```python
from build123d import *

# Parameters (mm, degrees)
SKETCH1_W           = 310
SKETCH1_H           = 120
SKETCH1_R           = 2.5
BOSS_EXTRUDE1_DEPTH = 3
CUT_EXTRUDE1_REACH  = 168.235
SKETCH2_R           = 12.5


with BuildPart() as part:
    # Sketch1 → Boss-Extrude1 (new body)
    with BuildSketch(Plane(origin=(0, 0, 0), x_dir=(1, 0, 0), z_dir=(0, 1, 0))):
        Rectangle(SKETCH1_W, SKETCH1_H)
        with Locations(Location((-125, 47, 0), (0, 0, 270))):
            Circle(SKETCH1_R, mode=Mode.SUBTRACT)
        with Locations(Location((125, 47, 0), (0, 0, 90))):
            Circle(SKETCH1_R, mode=Mode.SUBTRACT)
        with Locations(Location((125, -47, 0), (0, 0, 270))):
            Circle(SKETCH1_R, mode=Mode.SUBTRACT)
        with Locations(Location((-125, -47, 0), (0, 0, 90))):
            Circle(SKETCH1_R, mode=Mode.SUBTRACT)
    extrude(amount=BOSS_EXTRUDE1_DEPTH)

    # Sketch2 → Cut-Extrude1 (cut, up to next)
    with BuildSketch(Plane.XZ, mode=Mode.PRIVATE) as cut_extrude1_sk1:
        with Locations((155, -20)):
            Circle(SKETCH2_R)
    cut_extrude1_tool1 = extrude(cut_extrude1_sk1.sketch, amount=-CUT_EXTRUDE1_REACH, mode=Mode.PRIVATE) & part.part
    add(cut_extrude1_tool1.solids().sort_by_distance((155, 0, -20))[0], mode=Mode.SUBTRACT)


solid = part.part
```
Model file for the job. Use its own axes, mm. Give positions to 0.01 mm unless a question says otherwise; leave off trailing zeros. Loops run counter-clockwise (first coordinate to the right, second up) from the corner with the lowest first, then second, coordinate; pieces in that order, holes last. Notation, with made-up numbers: (-12.5, 65.5) -> (25.5, 65.5) arc R18 cw to (25.5, 83.5) -> close; hole circle Ø8 at (18.5, 55). An arc over 180 degrees is marked (long way). Use CSV: the item, a comma, the result in double quotes. Start each with the question number.
1) Mould opens along Z. For faces 1 (the cylindrical face through (-122.52, 1.48, -47.33)), 2 (the flat face through (-2, 0, -1)) say: released by +Z, released by -Z, zero draft, split by the parting line, or undercut.
2) Flat gauge pins, fed straight in: pin 1 Ø8 at (x, z) = (125, -47) entering from -Y; pin 2 Ø4.5 at (x, z) = (-125, 47) entering from +Y. Where does each tip first touch, or does it go through?
3) Slice it at A-A on z = -20. Give the cut face in (x, y).
4) Wall check: line 1 (X direction, y = 0.8, z = 47); line 2 (X direction, y = 2.7, z = -45). Give the ranges that are in metal, low to high.
Computed values:
1,face 1,"undercut"
1,face 2,"zero draft"
2,pin 1,"stops at y = 0"
2,pin 2,"passes through"
3,outline,"(-155, 0) -> (142.5, 0) -> (142.5, 3) -> (-155, 3) -> close"
4,line 1,"x = -155 to -127.5, -122.5 to 122.5, 127.5 to 155"
4,line 2,"x = -155 to -126.5, -123.5 to 123.5, 126.5 to 155"
